The model under review builds one solid part; all positions refer to its coordinate system, in mm. A direction names the side the tool comes from. Give positions to 0.01 mm unless a question says otherwise; leave off trailing zeros. Order: outer loops, then holes, each group sorted by start corner. A loop starts at its lowest first (then second) coordinate and runs counter-clockwise, first axis right, second up.
```python
from build123d import *

# Parameters (mm, degrees)
F1_DEPTH  = 8
F3_W      = 8
F3_H      = 8
F3_R      = 2.4
F4_DEPTH  = 1.7
F5_R      = 2.4
F6_DEPTH  = 1.7
F14_W     = 33.3092473447
F14_H     = 24.2573712021
F15_DEPTH = 16.002


with BuildPart() as f1:
    # F0 (on Front) → F1 (new body)
    with BuildSketch(Plane.XZ):
        Polygon((-2.4, 9.6), (-4, 9.6), (-4, 0), (4, 0), (4, 9.6), (2.4, 9.6), (2.4, 11.3), (-2.4, 11.3), align=None)
    extrude(amount=F1_DEPTH)

    # F3 (on plane+point) → F4 (cut, through all)
    with BuildSketch(Plane.XY.offset(11.3)):
        with Locations((0, -4)):
            Rectangle(F3_W, F3_H)
        with Locations((0, -4)):
            Circle(F3_R, mode=Mode.SUBTRACT)
    extrude(amount=-F4_DEPTH, mode=Mode.SUBTRACT)

    # F5 (on Top) → F6 (cut)
    with BuildSketch(Plane.XY):
        with Locations((0, -4)):
            Circle(F5_R)
    extrude(amount=F6_DEPTH, mode=Mode.SUBTRACT)

    # F8: F1 across plane


with BuildPart() as f1_1:
    add(f1.part)
    add(f1.part.mirror(Plane.YZ.offset(4)))

    # F9: F1 across plane


with BuildPart() as f1_2:
    add(f1_1.part)
    add(f1_1.part.mirror(Plane.XZ))

    # F11: F1 across plane


with BuildPart() as f1_3:
    add(f1_2.part)
    add(f1_2.part.mirror(Plane.YZ.offset(12)))

    # F12: F1 across face


with BuildPart() as f1_4:
    add(f1_3.part)
    add(f1_3.part.mirror(Plane(origin=(28, 0, 4.8), x_dir=(0, 1, 0), z_dir=(1, 0, 0))))

    # F14 (on offset) → F15 (cut)
    with BuildSketch(Plane.YZ.offset(60)):
        with Locations((2.0649190992, 4.5698834583)):
            Rectangle(F14_W, F14_H)
    extrude(amount=-F15_DEPTH, mode=Mode.SUBTRACT)


solid = f1_4.part
```
1. For faces 5 (the cylindrical face through (1.29, -1.976, 10.462)), 6 (the flat face through (0, -4, 11.3)), 7 (the cylindrical face through (34.217, -4.919, 0.838)), list the 3-axis set-ups (+Z, -Z, +X, -X, +Y, -Y) from which the entire face can be reached by the end or side of a thin tool; tool diameter is ignored.
2. To check wall thickness, follow line 1 (Y direction, x = 8, z = 0.85); line 2 (Y direction, x = 8.5, z = 1); line 3 (Z direction, x = 38, y = -2.75). State the ranges of each line that lie inside material, in increasing order.
3. Draft analysis for pull direction X (two halves, no side actions). For faces 1 (the cylindrical face through (1.29, 1.976, 10.462)), 2 (the cylindrical face through (42.398, -3.894, 10.462)), 3 (the flat face through (8, 4, 11.3)), 4 (the flat face through (-4, 0, 5)), state which applies: pulls with the +X half, pulls with the -X half, needs draft (parallel to the pull), parting line crosses it, or undercut.
4. Take a section at B-B (y = 0.5). Write out the cut boundary in (x, z), and give its area (3 significant figures).
5. Insertion check: pin 1 (5.5 mm diameter, centred on x = 31.5, y = -4, fed in from -Z); pin 2 (3 mm diameter, centred on x = 8, y = -4, fed in from -Z). Each pin has a flat end and moves straight along its axis. Give the tip position at first contact, or say it passes through.
6. Take a section at A-A (x = 24). Write out the cut boundary in (y, z).
Answer:
1. face 5: +Z
1. face 6: +Z, +X, -X, +Y, -Y
1. face 7: -Z
2. line 1: y = -8 to -6.4, -1.6 to 1.6, 6.4 to 8
2. line 2: y = -8 to -6.35, -1.65 to 1.65, 6.35 to 8
2. line 3: z = 1.7 to 11.3
3. face 1: undercut
3. face 2: undercut
3. face 3: needs draft
3. face 4: pulls with the -X half
4. outline: (-4, 0) - (44, 0) - (44, 9.6) - (-4, 9.6) - close
4. area: 461 mm2
5. pin 1: stops at z = 0
5. pin 2: stops at z = 1.7
6. outline: (-8, 0) - (-6.4, 0) - (-6.4, 1.7) - (-1.6, 1.7) - (-1.6, 0) - (1.6, 0) - (1.6, 1.7) - (6.4, 1.7) - (6.4, 0) - (8, 0) - (8, 9.6) - (6.4, 9.6) - (6.4, 11.3) - (1.6, 11.3) - (1.6, 9.6) - (-1.6, 9.6) - (-1.6, 11.3) - (-6.4, 11.3) - (-6.4, 9.6) - (-8, 9.6) - close
